Check sheet for the drawn part. Datum: minimum x, y, z corner. Units: mm. Coordinates: 2 decimals unless noted, no trailing zeros. Loops run counter-clockwise (first coordinate to the right, second up) from the corner with the lowest first, then second, coordinate; pieces in that order, holes last.
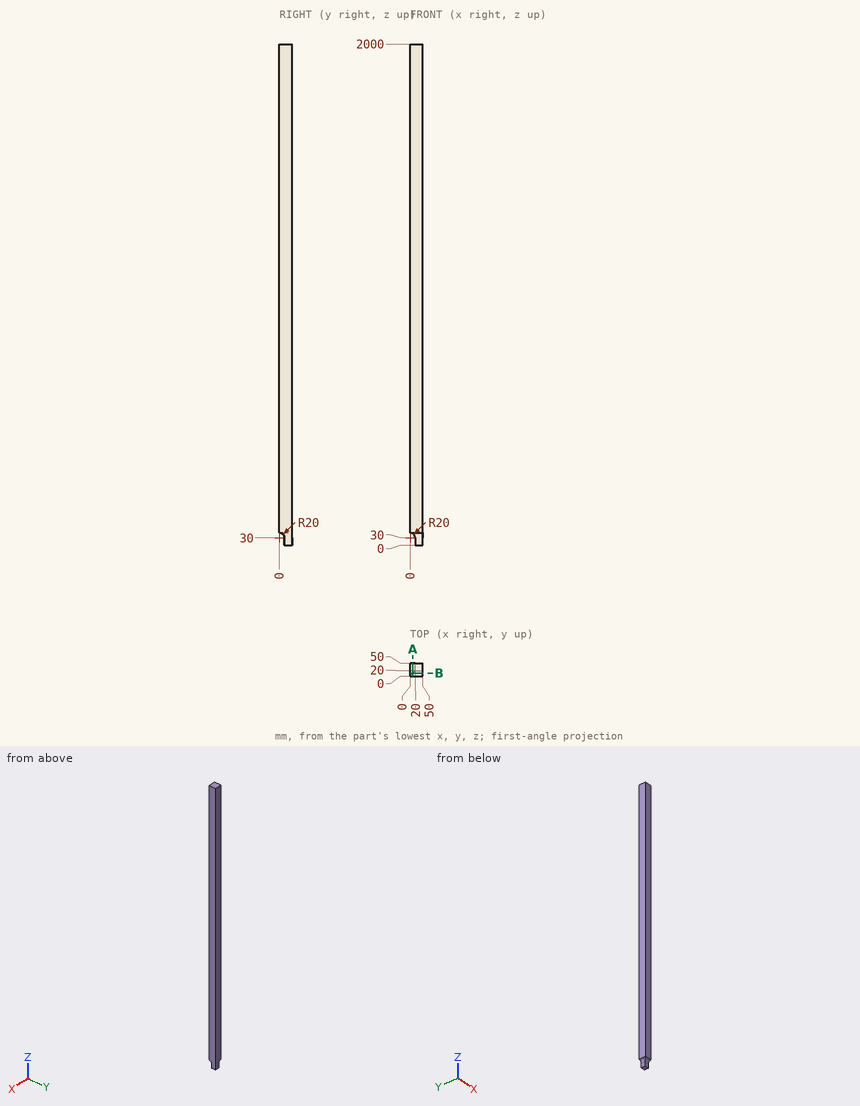
(1) Gauge pin test, flat ends, axial feed: pin 1 Ø8 at (y, z) = (39, 1057.5) entering from -X; pin 2 Ø2 at (x, y) = (29.5, 8) entering from -Z; pin 3 Ø15 at (x, z) = (38, 10.5) entering from -Y. Record the tip position at first contact, or that the pin passes through.
Findings:
pin 1: stops at x = 0
pin 2: stops at z = 47.86
pin 3: stops at y = 20
(2) Scan lines: L1, parallel to Z at x = 39, y = 4; L2, parallel to Z at x = 39, y = 9. Record each from-to range of solid material in increasing order.
Findings:
L1: z = 49.6 to 2000
L2: z = 47.86 to 2000
(3) Sectioned sample at B-B on y = 11.5. Record the cut outline in (x, z), and give its area (3 significant figures).
Findings:
outline: (0, 50) arc R20 cw to (11.5, 46.36) - (50, 46.36) - (50, 2000) - (0, 2000) - close
area: 97,700 mm2
(4) Sectioned sample at A-A on x = 11. Record the cut outline in (y, z), and give its area (3 significant figures).
Findings:
outline: (0, 50) arc R20 cw to (11, 46.7) - (50, 46.7) - (50, 2000) - (0, 2000) - close
area: 97,600 mm2
